Read the model definition and answer for the solid it produces. Units are mm, in the model's axes. Face numbers are marked on the shaded views. A direction names the side the tool comes from. Give positions to 0.01 mm unless a question says otherwise; leave off trailing zeros. Write each loop counter-clockwise with the first axis right and the second up, starting at its lowest first coordinate (ties: lowest second). Pieces come first, ordered by that corner, then holes. Notation, with made-up numbers: (7, -4.75) -> (33, -4.75) arc R12 cw to (33, 10.25) -> close; hole circle Ø8 at (59.25, 73). An arc over 180 degrees is marked (long way). Answer as CSV lines item,"result". Start each with the question number.
1. The part is cut by section C-C, the plane z = -2.5. Give the number of separate pieces and of enclosed holes in the cut face, and give its area (3 significant figures).
2. Given pin 1 (3 mm diameter, centred on x = 0, y = -11, fed in from +Z); pin 2 (0.8 mm diameter, centred on x = -0.5, z = 0.5, fed in from -Y); pin 3 (1.8 mm diameter, centred on x = -0.5, y = 8, fed in from +Z); pin 4 (1 mm diameter, centred on x = 0.5, y = 12, fed in from +Z), each flat-ended and moving along its own axis, determine where each tip first touches the part or whether it passes through.
3. The part is cut by section B-B, the plane y = 0. Determine the outline of the cut face in (x, z).
4. For a pull along Y with two mould halves and no side action, classify the marked faces 4 and 5 as pulls with the +Y half, pulls with the -Y half, needs draft (parallel to the pull), parting line crosses it, or undercut.
5. A tool of negligible diameter and unlimited length cuts with its end or side. For the marked faces 1, 2 and 3, from which of +Z, -Z, +X, -X, +Y, -Y can it reach the whole face along a straight path? Write none if from no direction.
6. Find the intervals of material crossed by line 1 (Z direction, x = 0, y = 0); line 2 (X direction, y = -10, z = 10.5); line 3 (Z direction, x = -2, y = -1), in increasing order.
7. The part is cut by section A-A, the plane x = 0. Determine the outline of the cut face in (y, z).
Autodesk Inventor part; units mm, degrees
ref_plane "body_screw_XY" through (0, -10, 5) normal (0, 0, 1) x (1, 0, 0)
ref_plane "body_screw_YZ" through (0, -10, 5) normal (1, 0, 0) x (0, 1, 0)
ref_plane "body_screw_ZX" through (0, -10, 5) normal (0, 1, 0) x (0, 0, 1)
sketch "Sketch_1" plane through (0, 0, 0) normal (0, 0, 1) x (1, 0, 0)
  line L0 (4, 0) -> (-4, 0)
  line L1 (-4, 14.5) -> (-4, 6.5)
  line L2 (-4, 6.5) -> (-3.5, 6)
  line L3 (-3.5, 6) -> (3.5, 6)
  line L4 (3.5, 6) -> (4, 6.5)
  line L5 (4, 6.5) -> (4, 14.5)
  line L6 (4, 14.5) -> (3.5, 15)
  line L7 (3.5, 15) -> (-3.5, 15)
  line L8 (-3.5, 15) -> (-4, 14.5)
revolve "Revolution1" add sketch "Sketch_1" angle 360 about axis through (4, 0, 0) along (1, 0, 0)
sketch "Sketch_2" plane through (0, 0, 0) normal (1, 0, 0) x (0, 1, 0)
  line L0 (-15, 0.75) -> (-15, -0.75)
  line L1 (-15, -0.75) -> (9.5, -0.75)
  line L2 (9.5, -0.75) -> (9.5, 0.75)
  line L3 (9.5, 0.75) -> (-15, 0.75)
extrude "Extrusion1" cut sketch "Sketch_2" along normal mid plane 8
sketch "Sketch_3" plane through (0, 0, 0) normal (1, 0, 0) x (0, 1, 0)
  line L0 (-10, 15) -> (-10, 0)
  line L1 (-10, 0) -> (-11.7, 0)
  line L2 (-11.7, 0) -> (-11.7, 5)
  line L3 (-11.7, 5) -> (-13, 5)
  line L4 (-13, 5) -> (-13, 15)
  line L5 (-13, 15) -> (-10, 15)
  line L6 (-10, 15) -> (-10, 0)
revolve "Revolution2" cut sketch "Sketch_3" angle 360 about axis through (0, -10, 15) along (0, 0, 1)
sketch "Sketch_4" plane through (0, 0, 0) normal (1, 0, 0) x (0, 1, 0)
  line L0 (-10, -15.75) -> (-10, -0.75)
  line L1 (-10, -0.75) -> (-8.5, -0.75)
  line L2 (-8.5, -0.75) -> (-8.7705, -1.0205)
  line L3 (-8.7705, -1.0205) -> (-8.7705, -15.75)
  line L4 (-8.7705, -15.75) -> (-10, -15.75)
  line L5 (-10, -15.75) -> (-10, -0.75)
revolve "Revolution3" cut sketch "Sketch_4" angle 360 about axis through (0, -10, -15.75) along (0, 0, -1)
thread "Thread1"
sketch "Sketch_7" plane through (0, 0, 0) normal (1, 0, 0) x (0, 1, 0)
  circle A0 centre (0, -11) radius 2.75
extrude "Extrusion2" cut sketch "Sketch_7" along normal mid plane 16
sketch "Sketch_8" plane through (0, 0, 0) normal (1, 0, 0) x (0, 1, 0)
  circle A0 centre (0, 11) radius 2.75
extrude "Extrusion3" cut sketch "Sketch_8" along normal mid plane 16
ref_plane "body_screw_XY" through (0, -10, 5) normal (0, 0, 1) x (1, 0, 0)
ref_plane "body_screw_YZ" through (0, -10, 5) normal (1, 0, 0) x (0, 1, 0)
ref_plane "body_screw_ZX" through (0, -10, 5) normal (0, 1, 0) x (0, 0, 1)
properties part number "SSCSM12-8b"
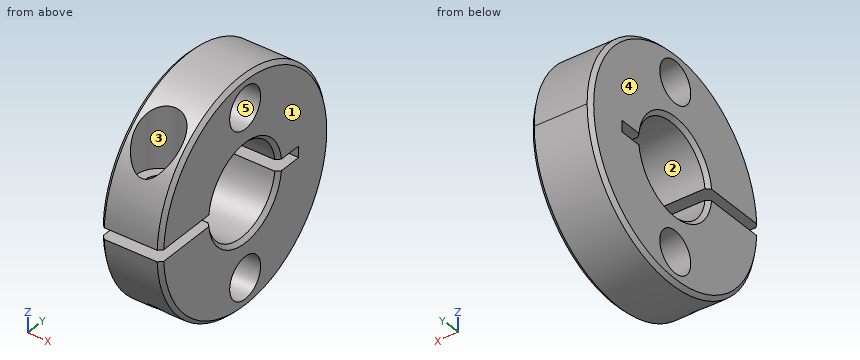
Results found:
1,separate pieces,"2"
1,enclosed holes,"1"
1,area,"144 mm²"
2,pin 1,"stops at z = 5"
2,pin 2,"stops at y = -14.98"
2,pin 3,"stops at z = 13.21"
2,pin 4,"stops at z = 9.63"
3,outline,"(-4, -14.5) -> (-3.5, -15) -> (3.5, -15) -> (4, -14.5) -> (4, -13.75) -> (-4, -13.75) -> close; (-4, -8.25) -> (4, -8.25) -> (4, -6.5) -> (3.5, -6) -> (-3.5, -6) -> (-4, -6.5) -> close; (-4, 6.5) -> (-3.5, 6) -> (3.5, 6) -> (4, 6.5) -> (4, 8.25) -> (-4, 8.25) -> close; (-4, 13.75) -> (4, 13.75) -> (4, 14.5) -> (3.5, 15) -> (-3.5, 15) -> (-4, 14.5) -> close"
4,face 4,"needs draft"
4,face 5,"undercut"
5,face 1,"+Z, -Z, +X, +Y, -Y"
5,face 2,"+X, -X"
5,face 3,"+Z"
6,line 1,"z = -15 to -13.75, -8.25 to -6, 6 to 8.25, 13.75 to 15"
6,line 2,"x = -4 to -3, 3 to 4"
6,line 3,"z = -14.97 to -13.56, -8.44 to -5.92, 5.92 to 8.44, 13.56 to 14.97"
7,outline,"(-14.98, -0.75) arc R15 ccw to (-11.23, -9.94) -> (-11.23, -1.02) -> (-11.5, -0.75) -> close; (-14.98, 0.75) -> (-11.7, 0.75) -> (-11.7, 5) -> (-13, 5) -> (-13, 7.48) arc R15 ccw to start; (-8.77, -12.17) arc R15 ccw (long way) to (-7, 13.27) -> (-7, 5) -> (-8.3, 5) -> (-8.3, 0.75) -> (-5.95, 0.75) arc R6 cw to (5.95, 0.75) -> (9.5, 0.75) -> (9.5, -0.75) -> (5.95, -0.75) arc R6 cw to (-5.95, -0.75) -> (-8.5, -0.75) -> (-8.77, -1.02) -> close; hole circle Ø5.5 at (0, -11); hole circle Ø5.5 at (0, 11)"
